Verification items for the finished model (mm, model axes). Give positions to 0.01 mm unless a question says otherwise; leave off trailing zeros. Write each loop counter-clockwise with the first axis right and the second up, starting at its lowest first coordinate (ties: lowest second). Pieces come first, ordered by that corner, then holes.
from build123d import *

# Parameters (mm, degrees)
CROQUIS1_W              = 222
CROQUIS1_H              = 18
CROQUIS1_R              = 1
CROQUIS1_R_2            = 6.5
CROQUIS1_W_2            = 3.5
CROQUIS1_H_2            = 10
SALIENTE_EXTRUIR1_DEPTH = 3
CROQUIS2_W              = 20
CROQUIS2_H              = 3
SALIENTE_EXTRUIR2_DEPTH = 3
CROQUIS3_W              = 3
CROQUIS3_H              = 10
SALIENTE_EXTRUIR3_DEPTH = 3


with BuildPart() as part:
    # Croquis1 → Saliente-Extruir1 (new body)
    with BuildSketch(Plane.XY):
        Rectangle(CROQUIS1_W, CROQUIS1_H)
        with Locations((-5, 5)):
            Circle(CROQUIS1_R, mode=Mode.SUBTRACT)
        with Locations(Location((5, 5, 0), (0, 0, 180))):
            Circle(CROQUIS1_R, mode=Mode.SUBTRACT)
        with Locations((-61.5, 0)):
            Circle(CROQUIS1_R_2, mode=Mode.SUBTRACT)
        with Locations(Location((61.5, 0, 0), (0, 0, 180))):
            Circle(CROQUIS1_R_2, mode=Mode.SUBTRACT)
        with Locations((32.25, 0)):
            Rectangle(CROQUIS1_W_2, CROQUIS1_H_2, mode=Mode.SUBTRACT)
        with Locations((-32.25, 0)):
            Rectangle(CROQUIS1_W_2, CROQUIS1_H_2, mode=Mode.SUBTRACT)
    extrude(amount=SALIENTE_EXTRUIR1_DEPTH)

    # Croquis2 → Saliente-Extruir2 (add)
    with BuildSketch(Plane(origin=(0, 9, 0), x_dir=(1, 0, 0), z_dir=(0, 1, 0))):
        with Locations((-65, -1.5)):
            Rectangle(CROQUIS2_W, CROQUIS2_H)
        with Locations((0, -1.5)):
            Rectangle(CROQUIS2_W, CROQUIS2_H)
        with Locations((65, -1.5)):
            Rectangle(CROQUIS2_W, CROQUIS2_H)
    extrude(amount=SALIENTE_EXTRUIR2_DEPTH)

    # Croquis3 → Saliente-Extruir3 (add)
    with BuildSketch(Plane(origin=(111, 0, 0), x_dir=(0, 0, -1), z_dir=(1, 0, 0))):
        with Locations((-1.5, -3.45)):
            Rectangle(CROQUIS3_W, CROQUIS3_H)
    saliente_extruir3 = extrude(amount=SALIENTE_EXTRUIR3_DEPTH)

    # Simetría1: Saliente-Extruir3 across plane
    add(saliente_extruir3.mirror(Plane(origin=(0, 0, 0), x_dir=(0, 0, 1), z_dir=(1, 0, 0))))


solid = part.part
Item 1: Scan lines: line 1 along X through (y, z) = (10, 2.9); line 2 along X through (y, z) = (-0.5, 1.3); line 3 along Y through (x, z) = (5, 2.45). Record each from-to range of solid material in increasing order.
Answer key:
line 1: x = -75 to -55, -10 to 10, 55 to 75
line 2: x = -114 to -67.98, -55.02 to -34, -30.5 to 30.5, 34 to 55.02, 67.98 to 114
line 3: y = -9 to 4, 6 to 12
Item 2: Sectioned sample at B-B on x = 59. Record the cut outline in (y, z).
Answer key:
outline: (-9, 0) - (-6, 0) - (-6, 3) - (-9, 3) - close; (6, 0) - (12, 0) - (12, 3) - (6, 3) - close
Item 3: Release check for a two-part mould opening along X. For faces 1 (the face through (-55.3, 1.95, 1.48)), 2 (the face through (55.3, -1.95, 1.48)), 3 (the face through (-2, 2, 3)) record: released by +X, released by -X, zero draft, split by the parting line, or undercut.
Answer key:
face 1: undercut
face 2: undercut
face 3: zero draft
Item 4: Depth check by flat-ended pin: pin 1 (10 mm diameter, centred on x = -46, y = -2, fed in from -Z); pin 2 (1.5 mm diameter, centred on x = 113, z = 1, fed in from +Y); pin 3 (0.9 mm diameter, centred on y = 10, z = 1, fed in from +X); pin 4 (0.9 mm diameter, centred on x = -101.5, z = 2, fed in from +Y). Enter the tip coordinate at first touch or a pass-through.
Answer key:
pin 1: stops at z = 0
pin 2: stops at y = 1.55
pin 3: stops at x = 75
pin 4: stops at y = 9
Item 5: Sectioned sample at A-A on x = -61.5. Record the cut outline in (y, z).
Answer key:
outline: (-9, 0) - (-6.5, 0) - (-6.5, 3) - (-9, 3) - close; (6.5, 0) - (12, 0) - (12, 3) - (6.5, 3) - close
Item 6: Sectioned sample at C-C on z = 1.45. State how many separate pieces and enclosed holes the cut face has, then the cut area to 3 significant figures.
Answer key:
separate pieces: 1
enclosed holes: 6
area: 3,890 mm2
